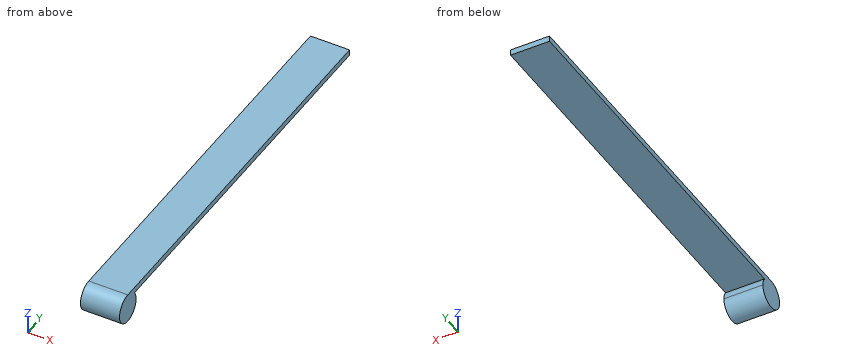
```python
from build123d import *

# Parameters (mm, degrees)
F1_DEPTH = 20


with BuildPart() as f1:
    # F0 (on Right) → F1 (new body)
    with BuildSketch(Plane.YZ):
        with BuildLine():
            Line((200, 7.5), (0, 7.5))
            ThreePointArc((0, 7.5), (3.354102, 6.708204), (6, 4.5))
            Line((6, 4.5), (200, 4.5))
            Line((200, 4.5), (200, 7.5))
        make_face()
        with BuildLine():
            ThreePointArc((6, 4.5), (3.354102, 6.708204), (0, 7.5))
            Line((0, 7.5), (0, 4.5))
            Line((0, 4.5), (6, 4.5))
        make_face()
        with BuildLine():
            Line((0, 4.5), (0, 7.5))
            ThreePointArc((0, 7.5), (-5.303301, -5.303301), (7.5, 0))
            ThreePointArc((7.5, 0), (7.115125, 2.371708), (6, 4.5))
            Line((6, 4.5), (0, 4.5))
        make_face()
    extrude(amount=F1_DEPTH)


solid = f1.part
```
Design review of the part built by this model. Coordinates are the model's own, in mm. Coordinates: 2 decimals unless noted, no trailing zeros. Write each loop counter-clockwise with the first axis right and the second up, starting at its lowest first coordinate (ties: lowest second). Pieces come first, ordered by that corner, then holes.
1) Add section B-B (z = -4). Write out the cut boundary in (x, y).
2) Add section A-A (x = 18.25). Write out the cut boundary in (y, z).
3) Insertion check: pin 1 (1 mm diameter, centred on x = 4, y = 119, fed in from -Z); pin 2 (3 mm diameter, centred on x = 7, z = 4, fed in from -Y); pin 3 (1 mm diameter, centred on x = 9, z = 5, fed in from -Y). Each pin has a flat end and moves straight along its axis. Give the tip position at first contact, or say it passes through.
4) To check wall thickness, follow L1, parallel to Z at x = 11, y = 8.5; L2, parallel to Y at x = 11.75, z = -0.25; L3, parallel to Y at x = 11.75, z = 1.5. State the ranges of each line that lie inside material, in increasing order.
Check result:
1. outline: (0, -6.34) - (20, -6.34) - (20, 6.34) - (0, 6.34) - close
2. outline: (0, 7.5) arc R7.5 ccw (long way) to (7.5, 0) arc R7.5 ccw to (6, 4.5) - (200, 4.5) - (200, 7.5) - close
3. pin 1: stops at z = 4.5
3. pin 2: stops at y = -7.07
3. pin 3: stops at y = -6
4. L1: z = 4.5 to 7.5
4. L2: y = -7.5 to 7.5
4. L3: y = -7.35 to 7.35
